Drawing for the job (mm, zero at the part's lowest x, y, z). A direction names the side the tool comes from. Give positions to 0.01 mm unless a question says otherwise; leave off trailing zeros. Write each loop counter-clockwise with the first axis right and the second up, starting at its lowest first coordinate (ties: lowest second). Pieces come first, ordered by that corner, then holes. Notation, with made-up numbers: M 64.25,30 L 121.25,30 A25 cw 121.25,53 Z; hole C -8.75,7 d2. An arc over 180 degrees is marked long. Use a Markdown table: item, result. Add a question column.
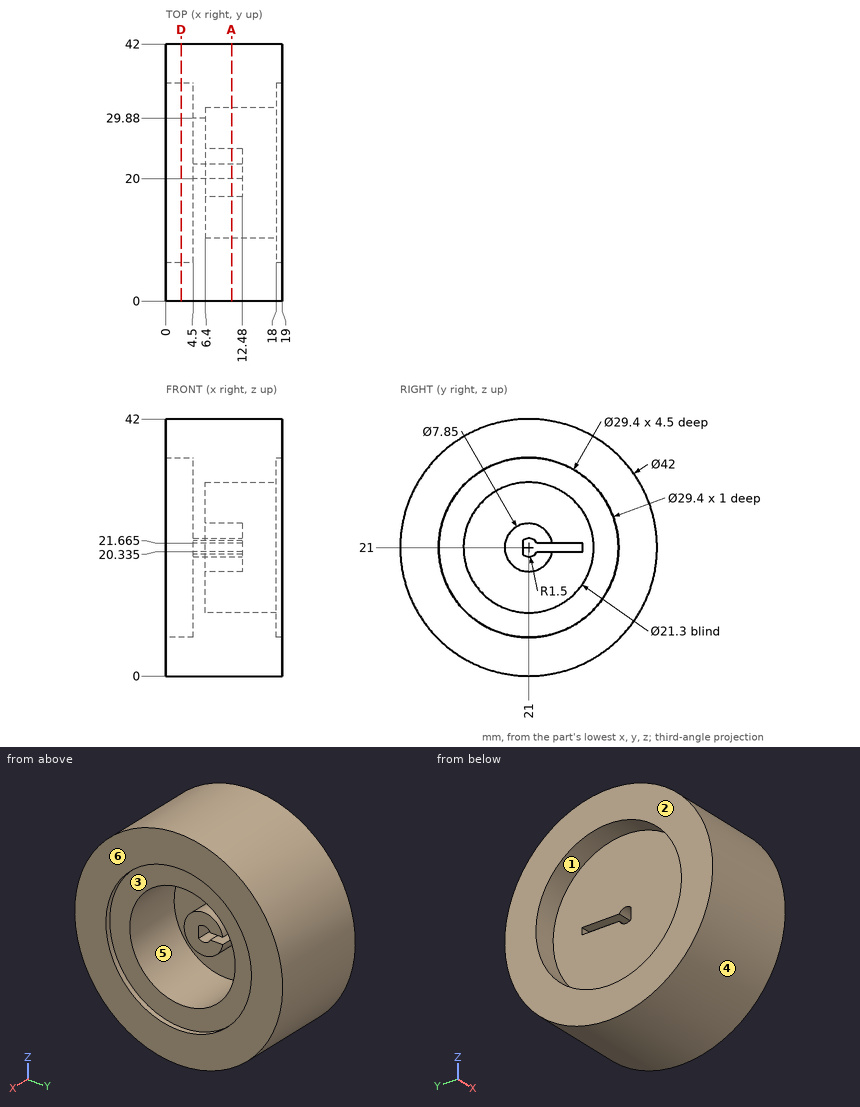
1. Cut at D-D (x = 2.5). Write the cut outline in (y, z).
2. Cut at A-A (x = 10.75). Give the number of separate pieces and of enclosed holes in the cut face, then the cut area to 3 significant figures.
3. Drill centre lines: probe 1 along Y at (x, z) = (2.05, 21); probe 2 along Y at (x, z) = (15.5, 21); probe 3 along Z at (x, y) = (7.5, 21.5) (1 decimal). Where is each one in solid material? Low to high. Write a range as [from, to].
4. Flat gauge pins, fed straight in: pin 1 (4 mm diameter, centred on x = 7.5, y = 25.5, fed in from -Z); pin 2 (2 mm diameter, centred on x = 4.5, y = 30, fed in from -Z); pin 3 (23.5 mm diameter, centred on y = 21, z = 21, fed in from -X). Where does each tip first touch, or does it go through?
5. Tool access for the marked faces 1, 2 and 3: list every direction of +Z, -Z, +X, -X, +Y, -Y with a clear straight run to the whole face (end or side of a thin tool).
6. Mould opens along Y. For the marked faces 4, 5 and 6 say: released by +Y, released by -Y, zero draft, split by the parting line, or undercut.
A:
| question | item | result |
|---|---|---|
| 1 | outline | C 21,21 d42; hole C 21,21 d29.4 |
| 2 | separate pieces | 2 |
| 2 | enclosed holes | 1 |
| 2 | area | 1,070 mm² |
| 3 | probe 1 | y = [0, 6.3], [35.7, 42] |
| 3 | probe 2 | y = [0, 10.35], [31.65, 42] |
| 3 | probe 3 | z = [0, 10.4], [17.1, 19.6], [22.4, 24.9], [31.6, 42] |
| 4 | pin 1 | stops at z = 0.15 |
| 4 | pin 2 | stops at z = 1.58 |
| 4 | pin 3 | stops at x = 4.5 |
| 5 | face 1 | -X |
| 5 | face 2 | +Z, -Z, -X, +Y, -Y |
| 5 | face 3 | +X |
| 6 | face 4 | split by the parting line |
| 6 | face 5 | undercut |
| 6 | face 6 | zero draft |
